The model under review builds one solid part; all positions refer to its coordinate system, in mm. A direction names the side the tool comes from. Coordinates: 2 decimals unless noted, no trailing zeros. Loops run counter-clockwise (first coordinate to the right, second up) from the corner with the lowest first, then second, coordinate; pieces in that order, holes last. Notation, with made-up numbers: (-33.5, -2) - (-21.5, -2) arc R16 ccw to (-21.5, 20) - close; hole circle Ø5 at (82.5, -24.5). An arc over 180 degrees is marked (long way). Use a Markdown table: item, result. Add a question column.
1) Clearance check with a flat-ended pin moving along its axis: pin 1 (2.5 mm diameter, centred on x = -0.5, y = 0.5, fed in from +Z). State where the tip first meets the part, or that it passes through.
2) The part is to be moulded in two halves that separate along X. For faces 4 (the flat face through (-7.9, 0, 5)), 5 (the flat face through (7.9, 0, 5)), 6 (the cylindrical face through (-0.702, -3.163, 5.181)), say which applies: pulls with the +X half, pulls with the -X half, needs draft (parallel to the pull), parting line crosses it, or undercut.
3) Add section A-A, the plane z = 8.5. Give the boundary of the cut face in (x, y) (3 decimals), and give its area (3 significant figures).
4) Add section D-D, the plane z = -0.25. Give the boundary of the cut face in (x, y) (3 decimals).
5) Add section B-B, the plane x = 0. Give the boundary of the cut face in (y, z) (3 decimals), and give its area (3 significant figures).
6) For faces 1 (the cylindrical face through (-3.421, -1.077, -1.035)), 2 (the flat face through (4, -3, -2.1)), 3 (the flat face through (-3, 2, 0.74)), list the 3-axis set-ups (+Z, -Z, +X, -X, +Y, -Y) from which the entire face can be reached by the end or side of a thin tool; tool diameter is ignored.
7) To check wall thickness, follow L1, parallel to Y at x = 0, z = 4.75 (3 decimals); L2, parallel to Y at x = -1.75, z = 3.5; L3, parallel to Y at x = -2.5, z = 3.25. State the ranges of each line that lie inside material, in increasing order. Write a range as [from, to].
```python
from build123d import *

# Parameters (mm, degrees)
F0_W     = 15.8
F0_H     = 15.8
F0_R     = 2.425
F1_DEPTH = 9.5
F2_DEPTH = 2.1
F3_W     = 13.32
F3_H     = 13.32
F3_R     = 3.24
F4_DEPTH = 8.76
F5_R     = 2.375
F6_DEPTH = 8.7


# Not quite as in the source:
# - a feature names something its author has since deleted; it is built from what else it names


with BuildPart() as f1:
    # F0 (on Top) → F1 (new body)
    with BuildSketch(Plane.XY):
        Rectangle(F0_W, F0_H)
        with Locations((-3.1053028645, -3.481)):
            Circle(F0_R, mode=Mode.SUBTRACT)
        with Locations((3.6446971353, -3.4810496163)):
            Circle(F0_R, mode=Mode.SUBTRACT)
        with Locations((-3.1053028647, 3.481)):
            Circle(F0_R, mode=Mode.SUBTRACT)
        with Locations((3.6446971353, 3.481)):
            Circle(F0_R, mode=Mode.SUBTRACT)
        with Locations((3.6446971353, -3.4810496163)):
            Circle(F0_R)
        with Locations((-3.1053028645, -3.481)):
            Circle(F0_R)
        with Locations((-3.1053028647, 3.481)):
            Circle(F0_R)
        with Locations((3.6446971353, 3.481)):
            Circle(F0_R)
    extrude(amount=F1_DEPTH)

    # F0 (on Top) → F2 (join)
    with BuildSketch(Plane.XY):
        with Locations((3.6446971353, 3.481)):
            Circle(F0_R)
        with Locations((-3.1053028647, 3.481)):
            Circle(F0_R)
        with Locations((-3.1053028645, -3.481)):
            Circle(F0_R)
        with Locations((3.6446971353, -3.4810496163)):
            Circle(F0_R)
    extrude(amount=-F2_DEPTH)

    # F3 (on face) → F4 (cut)
    with BuildSketch(Plane.XY.offset(9.5)):
        Rectangle(F3_W, F3_H)
        Circle(F3_R, mode=Mode.SUBTRACT)
    extrude(amount=-F4_DEPTH, mode=Mode.SUBTRACT)

    # F5 (on face) → F6 (cut)
    with BuildSketch(Plane.XY.offset(9.5)):
        Circle(F5_R)
    extrude(amount=-F6_DEPTH, mode=Mode.SUBTRACT)


solid = f1.part
```
From the geometry:
| question | item | result |
|---|---|---|
| 1 | pin 1 | stops at z = 0.8 |
| 2 | face 4 | pulls with the -X half |
| 2 | face 5 | pulls with the +X half |
| 2 | face 6 | undercut |
| 3 | outline | (-7.9, -7.9) - (7.9, -7.9) - (7.9, 7.9) - (-7.9, 7.9) - close; circle Ø6.48 at (0, 0); hole (-6.66, -6.66) - (6.66, -6.66) - (6.66, 6.66) - (-6.66, 6.66) - close; hole circle Ø4.75 at (0, 0) |
| 3 | area | 87.5 mm^2 |
| 4 | outline | circle Ø4.85 at (-3.105, -3.481); circle Ø4.85 at (-3.105, 3.481); circle Ø4.85 at (3.645, -3.481); circle Ø4.85 at (3.645, 3.481) |
| 5 | outline | (-7.9, 0) - (7.9, 0) - (7.9, 9.5) - (6.66, 9.5) - (6.66, 0.74) - (3.24, 0.74) - (3.24, 9.5) - (2.375, 9.5) - (2.375, 0.8) - (-2.375, 0.8) - (-2.375, 9.5) - (-3.24, 9.5) - (-3.24, 0.74) - (-6.66, 0.74) - (-6.66, 9.5) - (-7.9, 9.5) - close |
| 5 | area | 48.9 mm^2 |
| 6 | face 1 | -Z |
| 6 | face 2 | -Z, +X, -X, +Y, -Y |
| 6 | face 3 | +Z |
| 7 | L1 | y = [-7.9, -6.66], [-3.24, -2.375], [2.375, 3.24], [6.66, 7.9] |
| 7 | L2 | y = [-7.9, -6.66], [-2.73, -1.61], [1.61, 2.73], [6.66, 7.9] |
| 7 | L3 | y = [-7.9, -6.66], [-2.06, 2.06], [6.66, 7.9] |
